Verification items for this drawing (mm, ordinates from the low corner). A direction names the side the tool comes from. Coordinates: 2 decimals unless noted, no trailing zeros. Order: outer loops, then holes, each group sorted by start corner. A loop starts at its lowest first (then second) coordinate and runs counter-clockwise, first axis right, second up.
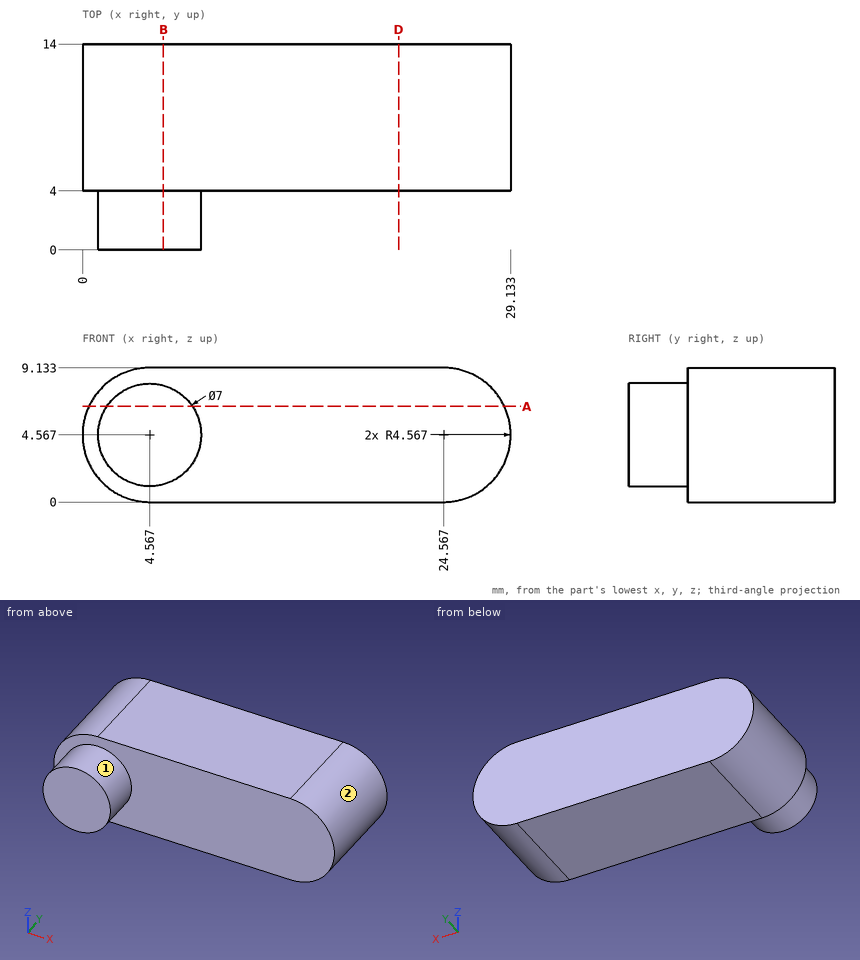
(1) Cross-section at B-B (x = 5.5). Enter the section's corners in (y, z).
Filled in:
outline: (0, 1.19) - (4, 1.19) - (4, 0) - (14, 0) - (14, 9.13) - (4, 9.13) - (4, 7.94) - (0, 7.94) - close
(2) Go/stop test with flat-tipped pins: P1, Ø2, axis at x = 10, z = 2, coming from the -Y side; P2, Ø1, axis at y = 11, z = 3, coming from the +X side. Record where each tip stops, or that it passes through.
Filled in:
P1: stops at y = 4
P2: stops at x = 29.01
(3) Thickness scan on probe 1 along Y at (x, z) = (7.5, 8.75); probe 2 along X at (y, z) = (8.25, 3.25) (1 decimal); probe 3 along X at (y, z) = (10.5, 5.5). Record the ranges inside material, lowest first.
Filled in:
probe 1: y = 4 to 14
probe 2: x = 0.2 to 28.9
probe 3: x = 0.1 to 29.04
(4) Cross-section at A-A (z = 6.5). Enter the section's corners in (x, y).
Filled in:
outline: (0.43, 4) - (1.65, 4) - (1.65, 0) - (7.48, 0) - (7.48, 4) - (28.7, 4) - (28.7, 14) - (0.43, 14) - close
(5) Cross-section at D-D (x = 21.5). Enter the section's corners in (y, z).
Filled in:
outline: (4, 0) - (14, 0) - (14, 9.13) - (4, 9.13) - close
(6) Tool access check on the marked faces 1 and 2. Record the directions out of +Z, -Z, +X, -X, +Y, -Y that give a thin tool (end or side, any length) a straight path to the whole face; none if there is none.
Filled in:
face 1: -Y
face 2: +X, +Y, -Y
